Read the model definition and answer for the solid it produces. Units are mm, in the model's axes. Face numbers are marked on the shaded views. A direction names the side the tool comes from. Coordinates: 2 decimals unless noted, no trailing zeros. Write each loop counter-clockwise with the first axis right and the second up, starting at its lowest first coordinate (ties: lowest second). Pieces come first, ordered by that corner, then holes.
(1) Find the intervals of material crossed by probe 1 along X at (y, z) = (-0.5, 0); probe 2 along Y at (x, z) = (2, -0.2); probe 3 along Z at (x, y) = (1.05, 1.25), in increasing order.
(2) Section A-A on y = 4.5 is taken. Write down the section's boundary in (x, z).
(3) Which of the six approach directions +Z, -Z, +X, -X, +Y, -Y give full straight-line access (tool end or side, diameter ignored) to the marked faces 4 and 5?
(4) Section C-C on y = -5.25 is taken. Write down the section's boundary in (x, z).
(5) Section D-D on z = 2.15 is taken. Write down the section's boundary in (x, y).
(6) The mould has two halves that part along Z. Classify the marked faces 1, 2 and 3: +Z half, -Z half, draft (parallel to the pull), parting line (faces both ways), or undercut.
(7) Section B-B on z = 0 is taken. Write down the section's boundary in (x, y).
from build123d import *

# Parameters (mm, degrees)
BOSS_EXTRUDE1_DEPTH = 6
SKETCH2_R           = 1.5
CUT_EXTRUDE1_DEPTH  = 8
SKETCH3_R           = 1.5
BOSS_EXTRUDE2_DEPTH = 3
CHAMFER2_SIZE       = 0.25


with BuildPart() as part:
    # Sketch1 → Boss-Extrude1 (new, symmetric)
    with BuildSketch(Plane(origin=(0, 0, 0), x_dir=(1, 0, 0), z_dir=(0, 1, 0))):
        Polygon((0, 2.886751346), (-2.5, 1.443375673), (-2.5, -1.443375673), (0, -2.886751346), (2.5, -1.443375673), (2.5, 1.443375673), align=None)
    extrude(amount=BOSS_EXTRUDE1_DEPTH, both=True)

    # Sketch2 → Cut-Extrude1 (cut)
    with BuildSketch(Plane(origin=(0, 6, 0), x_dir=(1, 0, 0), z_dir=(0, 1, 0))):
        with Locations(Location((0, 0, 0), (0, 0, 270))):
            Circle(SKETCH2_R)
    extrude(amount=-CUT_EXTRUDE1_DEPTH, mode=Mode.SUBTRACT)

    # Sketch3 → Boss-Extrude2 (add)
    with BuildSketch(Plane.XZ.offset(6)):
        with Locations(Location((0, 0, 0), (0, 0, 90))):
            Circle(SKETCH3_R)
    extrude(amount=BOSS_EXTRUDE2_DEPTH)

    # Chamfer2
    chamfer2_edges = [part.edges().sort_by_distance(p)[0] for p in [
        (0, 6, -1.5),
        (0, -9, -1.5),
    ]]
    chamfer(chamfer2_edges, length=CHAMFER2_SIZE)


solid = part.part
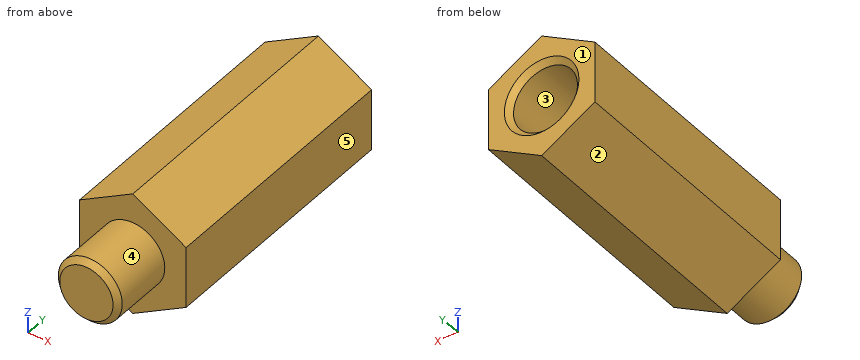
Response:
1. probe 1: x = -2.5 to -1.5, 1.5 to 2.5
1. probe 2: y = -6 to 6
1. probe 3: z = -2.28 to -1.07, 1.07 to 2.28
2. outline: (-2.5, -1.44) - (0, -2.89) - (2.5, -1.44) - (2.5, 1.44) - (0, 2.89) - (-2.5, 1.44) - close; hole circle Ø3 at (0, 0)
3. face 4: -Y
3. face 5: +Z, -Z, +X, +Y, -Y
4. outline: (-2.5, -1.44) - (0, -2.89) - (2.5, -1.44) - (2.5, 1.44) - (0, 2.89) - (-2.5, 1.44) - close
5. outline: (-1.28, -6) - (1.28, -6) - (1.28, 6) - (-1.28, 6) - close
6. face 1: draft
6. face 2: -Z half
6. face 3: undercut
7. outline: (-2.5, -6) - (-1.5, -6) - (-1.5, -8.75) - (-1.25, -9) - (1.25, -9) - (1.5, -8.75) - (1.5, -6) - (2.5, -6) - (2.5, 6) - (1.75, 6) - (1.5, 5.75) - (1.5, -2) - (-1.5, -2) - (-1.5, 5.75) - (-1.75, 6) - (-2.5, 6) - close
